Autodesk Inventor part; units mm, degrees
ref_plane "YZ Plane" through (0, 0, 0) normal (1, 0, 0) x (0, 1, 0)
ref_plane "XZ Plane" through (0, 0, 0) normal (0, 1, 0) x (-1, 0, 0)
ref_plane "XY Plane" through (0, 0, 0) normal (0, 0, 1) x (1, 0, 0)
sketch "スケッチ1" plane through (0, 0, 0) normal (1, 0, 0) x (0, 1, 0)
  circle A0 centre (0, 0) radius 9
  circle A1 centre (0, 0) radius 6.5
  dimension "d0" = 18
  dimension "d1" = 13
extrude "押し出し1" add sketch "スケッチ1" against normal blind 200
sketch "スケッチ2" plane through (0, 0, 0) normal (0, 1, 0) x (-1, 0, 0)
  point P0 (0, 0)
sketch "スケッチ3" plane through (0, 0, 0) normal (0, 0, 1) x (1, 0, 0)
  line L0 (0, 0) -> (0, 6)
  line L1 (0, 6.5) -> (0, -6.5)
  line L2 (0, 6) -> (-6, 6)
  line L3 (-6, 6) -> (-6, -6)
  line L4 (-6, -6) -> (0, -6)
  line L5 (0, -6) -> (0, 0)
  dimension "d4" = 6
  dimension "d5" = 6
  dimension "d6" = 12
extrude "押し出し2" cut sketch "スケッチ3" along normal mid plane 200
sketch "スケッチ4" plane through (0, 0, 0) normal (0, 0, 1) x (1, 0, 0)
  line L0 (-6, -6) -> (-6, 6)
  line L1 (0, 6) -> (-6, 6)
  circle A0 centre (-6, 0) radius 6
  point P0 (0, 0)
extrude "押し出し3" cut sketch "スケッチ4" along normal mid plane 200 contours A0 L0 picked at (-9.4508, 1.581)
sketch "スケッチ5" plane through (0, 0, 0) normal (0, 0, 1) x (1, 0, 0)
  circle A0 centre (-190, 0) radius 1.5
  point P0 (0, 0)
  dimension "d11" = 3
extrude "押し出し4" cut sketch "スケッチ5" along normal mid plane 200
thread "ねじ1"
thread "ねじ2"
properties part number "vp13_200" material "PVC 配管"
Read the model definition and answer for the solid it produces. Units are mm, in the model's axes. Round coordinates to 2 decimals unless told otherwise and drop trailing zeros. Loops run counter-clockwise (first coordinate to the right, second up) from the corner with the lowest first, then second, coordinate; pieces in that order, holes last.
Q1. Each of these flat-tipped pins is pushed along its axis until it touches: pin 1 (2 mm diameter, centred on x = -1.5, z = -5.5, fed in from +Y); pin 2 (4.5 mm diameter, centred on x = -2.5, z = 4, fed in from -Y); pin 3 (1 mm diameter, centred on y = 4.5, z = 1, fed in from +X); pin 4 (1 mm diameter, centred on x = -60.5, z = 6, fed in from -Y). Where does it stop, or does it pass through?
Q2. Section A-A on z = 0 is taken. Write down the section's boundary in (x, y), and give its area (3 significant figures).
Q3. Section B-B on x = -27 is taken. Write down the section's boundary in (y, z).
Q4. Consider probe 1 along Y at (x, z) = (-70, 0); probe 2 along X at (y, z) = (0, -7.4). Determine where each line is inside the solid, lowest interval first.
Q5. Determine the mould class of faces 1 (the face through (-98.6, -6.494, 0.286)), 2 (the face through (-12, 0, 7)), 3 (the face through (-98.6, -1.172, 8.923)), 4 (the face through (-200, 3, -6)) for opening direction Y: released by +Y, released by -Y, zero draft, split by the parting line, or undercut.
Output:
1. pin 1: stops at y = 7.79
1. pin 2: stops at y = -8.83
1. pin 3: passes through
1. pin 4: stops at y = -7.12
2. outline: (-200, -9) - (0, -9) - (0, -6.5) - (-200, -6.5) - close; (-200, 6.5) - (0, 6.5) - (0, 9) - (-200, 9) - close
2. area: 1,000 mm2
3. outline: circle Ø18 at (0, 0); hole circle Ø13 at (0, 0)
4. probe 1: y = -9 to -6.5, 6.5 to 9
4. probe 2: x = -200 to -191.5, -188.5 to -12
5. face 1: undercut
5. face 2: undercut
5. face 3: split by the parting line
5. face 4: zero draft
